Part model, mm, in its own coordinate system. Round coordinates to 2 decimals unless told otherwise and drop trailing zeros. Write each loop counter-clockwise with the first axis right and the second up, starting at its lowest first coordinate (ties: lowest second). Pieces come first, ordered by that corner, then holes.
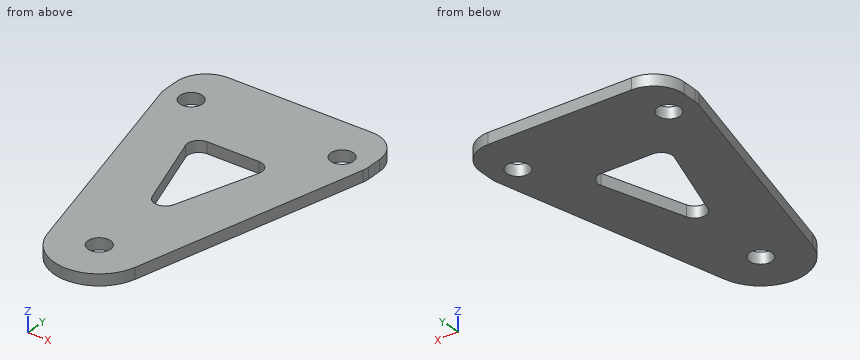
Autodesk Fusion 360 part; units mm, degrees
sketch "Sketch1" plane through (0, 0, 0) normal (0, 0, 1) x (1, 0, 0) in component "X Axis Support - Inside Support V2"
  line L0 (0, 0) -> (64, 0)
  line L1 (64, 0) -> (64, 84)
  line L2 (64, 84) -> (0, 84)
  line L3 (0, 84) -> (0, 0)
  dimension "d1" = 64
  dimension "d2" = 84
extrude "Extrude1" add sketch "Sketch1" along normal blind 3 in component "X Axis Support - Inside Support V2"
sketch "Sketch2" plane through (0, 0, 3) normal (0, 0, 1) x (-1, 0, 0) in component "X Axis Support - Inside Support V2"
  line L0 (0, -84) -> (0, 0)
  line L1 (0, 0) -> (-64, 0)
  line L2 (-64, 0) -> (-64, -84)
  line L3 (-64, -84) -> (0, -84)
  line L4 (-12, -84) -> (-12, 0) construction
  line L5 (-52, -84) -> (-52, 0) construction
  line L6 (0, -12) -> (-64, -12) construction
  line L7 (0, -72) -> (-64, -72) construction
  circle A0 centre (-12, -72) radius 12 construction
  circle A1 centre (-52, -72) radius 12 construction
  circle A2 centre (-12, -72) radius 3
  circle A3 centre (-52, -72) radius 3
  line L8 (0, -72) -> (0, 0)
  line L9 (0, 0) -> (-32, 0)
  line L10 (-32, 0) -> (-64, 0)
  line L11 (-64, 0) -> (-64, -72)
  circle A4 centre (-32, -12) radius 12
  circle A5 centre (-32, -12) radius 3
  line L12 (0, -26) -> (-64, -26) construction
  line L13 (-12, 0) -> (0, -26)
  line L14 (-52, 0) -> (-64, -26)
  line L15 (0, -85) -> (-64, -85) construction
  line L16 (-32, -85) -> (-32, 0) construction
  line L17 (-5.205, -70.3183) -> (-20.3514, -9.1171)
  line L18 (0, -60) -> (-64, -60) construction
  line L19 (0, -26) -> (-64, -26) construction
  line L20 (-21, -60) -> (-21, -26) construction
  line L21 (-43, -60) -> (-43, -26) construction
  line L22 (-21, -60) -> (-43, -60)
  line L23 (-32, -26) -> (-43, -60)
  line L24 (-32, -26) -> (-21, -60)
  circle A6 centre (-12, -72) radius 5 construction
  circle A7 centre (-52, -72) radius 5 construction
  circle A8 centre (-12, -72) radius 7
  circle A9 centre (-52, -72) radius 7
  line L25 (-58.795, -70.3183) -> (-43.6486, -9.1171)
  line L26 (-5, -72) -> (-5, -84)
  line L27 (-59, -72) -> (-59, -84)
  dimension "d8" = 12
  dimension "d13" = 24
  dimension "d14" = 24
  dimension "d16" = 6
  dimension "d17" = 6
  dimension "d40" = 60
  dimension "d53" = 24
  dimension "d55" = 6
  dimension "d57" = 26
  dimension "d234" = 13
  dimension "d238" = 20
  dimension "d241" = 20
  dimension "d242" = 60
  dimension "d243" = 14
  dimension "d244" = 11
  dimension "d245" = 11
  dimension "d248" = 10
  dimension "d249" = 10
  dimension "d250" = 14
  dimension "d251" = 14
extrude "Extrude2" cut sketch "Sketch2" against normal up to surface (3 mm away) contours L0 L1 L3 L8 L9 A4 L13 L17 A8 L26 | L0 L1 L8 L9 L13 | L1 L2 L3 L10 L11 A4 L14 A9 L25 L27 | L1 L2 L10 L11 L14 | A2 | A3 | A5 | L22 L23 L24 in component "X Axis Support - Inside Support V2"
fillet "Fillet11" radius 3 3 edges at (21, 60, 1.5) (43, 60, 1.5) (32, 26, 1.5) in component "X Axis Support - Inside Support V2"
fillet "Fillet11" radius 8 2 edges at (59, 84, 1.5) (5, 84, 1.5) in component "X Axis Support - Inside Support V2"
component "X Axis Support - Inside Support V2" placed x (1, 0, 0) y (0, 1, 0) z (0, 0, 1) at (0, 0, 0)
Q1. Cut at D-D on z = 1.85. Write the cut outline in (x, y) (3 decimals).
Values follow:
outline: (5, 72) arc R7 ccw to (5.205, 70.318) - (20.351, 9.117) arc R12 ccw to (43.649, 9.117) - (58.795, 70.318) arc R7 ccw to (59, 72) - (59, 76) arc R8 ccw to (51, 84) - (13, 84) arc R8 ccw to (5, 76) - close; hole circle Ø6 at (12, 72); hole (22.269, 56.077) - (29.146, 34.822) arc R3 ccw to (34.854, 34.822) - (41.731, 56.077) arc R3 ccw to (38.876, 60) - (25.124, 60) arc R3 ccw to start; hole circle Ø6 at (32, 12); hole circle Ø6 at (52, 72)
Q2. Drop flat-ended pins along their axis: pin 1 (5 mm diameter, centred on x = 12, y = 72, fed in from -Z); pin 2 (7 mm diameter, centred on x = 32, y = 12, fed in from +Z). Give the stop position or say it passes through.
Values follow:
pin 1: passes through
pin 2: stops at z = 3
Q3. Wall check: L1, parallel to X at y = 72, z = 1; L2, parallel to X at y = 73.5, z = 1.25; L3, parallel to X at y = 48, z = 0.45. Give the ranges that are in metal, low to high.
Values follow:
L1: x = 5 to 9, 15 to 49, 55 to 59
L2: x = 5 to 9.4, 14.6 to 49.4, 54.6 to 59
L3: x = 10.73 to 24.88, 39.12 to 53.27
Q4. Cut at B-B on x = 32. Write the cut outline in (y, z).
Values follow:
outline: (0, 0) - (9, 0) - (9, 3) - (0, 3) - close; (15, 0) - (32.75, 0) - (32.75, 3) - (15, 3) - close; (60, 0) - (84, 0) - (84, 3) - (60, 3) - close
Q5. Cut at A-A on y = 12. Write the cut outline in (x, z), plus the area to 3 significant figures.
Values follow:
outline: (19.64, 0) - (29, 0) - (29, 3) - (19.64, 3) - close; (35, 0) - (44.36, 0) - (44.36, 3) - (35, 3) - close
area: 56.2 mm2
Q6. Cut at C-C on x = 52. Write the cut outline in (y, z).
Values follow:
outline: (42.86, 0) - (69, 0) - (69, 3) - (42.86, 3) - close; (75, 0) - (83.94, 0) - (83.94, 3) - (75, 3) - close
